Geometry check sheet. Reference: drawing and pictorial views, mm from the part's lowest x, y, z. Give positions to 0.01 mm unless a question says otherwise; leave off trailing zeros. Loops run counter-clockwise (first coordinate to the right, second up) from the corner with the lowest first, then second, coordinate; pieces in that order, holes last. Notation, with made-up numbers: (-12.75, 37.25) -> (10.25, 37.25) arc R16 ccw to (10.25, 41.25) -> close; hole circle Ø10 at (31.25, 6). An arc over 180 degrees is marked (long way). One line per item, written item: value. Start each with the question number.
(1) Gauge pin test, flat ends, axial feed: pin 1 Ø1 at (x, z) = (19, 0.5) entering from +Y; pin 2 Ø1.5 at (y, z) = (50.5, 1) entering from +X. Record the tip position at first contact, or that the pin passes through.
(2) Sectioned sample at B-B, the plane z = 0.75. Record the cut outline in (x, y), then the cut area to 3 significant figures.
(3) Sectioned sample at C-C, the plane y = 60. Record the cut outline in (x, z), then the cut area to 3 significant figures.
(4) Sectioned sample at D-D, the plane x = 48.5. Record the cut outline in (y, z).
(5) Scan lines: line 1 along X through (y, z) = (14.5, 1.9) (1 decimal); line 2 along Y through (x, z) = (15.5, 2.1) (1 decimal); line 3 along X through (y, z) = (72.5, 0.9) (1 decimal). Record each from-to range of solid material in increasing order. Write a range as from..to.
(6) Sectioned sample at A-A, the plane y = 15. Record the cut outline in (x, z), then the cut area to 3 significant figures.
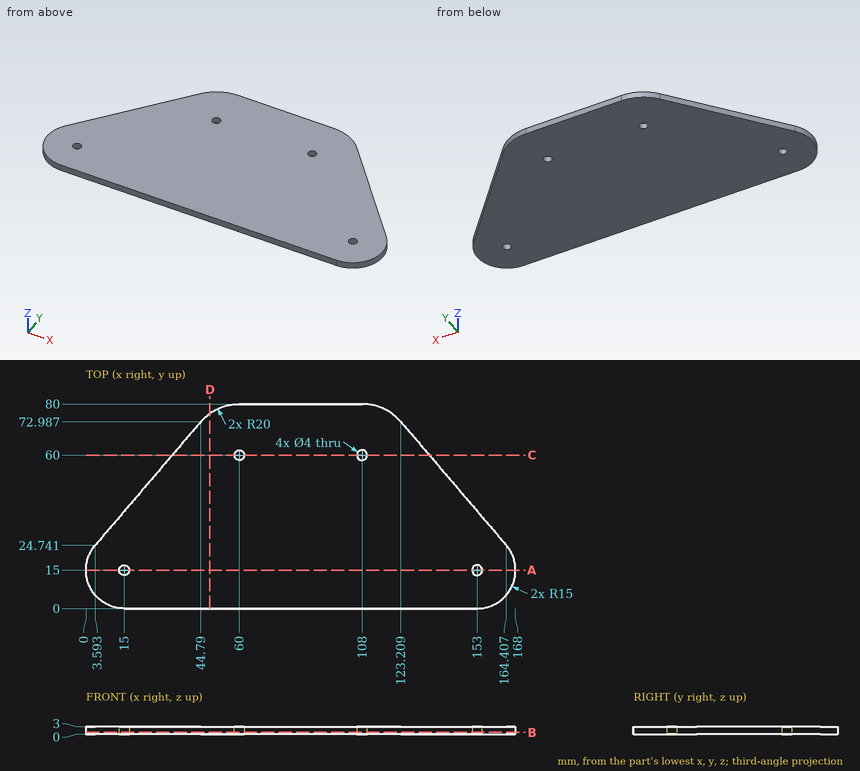
Calculated:
1. pin 1: stops at y = 43.37
1. pin 2: stops at x = 143.05
2. outline: (3.59, 24.74) arc R15 ccw to (15, 0) -> (153, 0) arc R15 ccw to (164.41, 24.74) -> (123.21, 72.99) arc R20 ccw to (108, 80) -> (60, 80) arc R20 ccw to (44.79, 72.99) -> close; hole circle Ø4 at (15, 15); hole circle Ø4 at (60, 60); hole circle Ø4 at (108, 60); hole circle Ø4 at (153, 15)
2. area: 10,200 mm2
3. outline: (33.7, 0) -> (58, 0) -> (58, 3) -> (33.7, 3) -> close; (62, 0) -> (106, 0) -> (106, 3) -> (62, 3) -> close; (110, 0) -> (134.3, 0) -> (134.3, 3) -> (110, 3) -> close
3. area: 278 mm2
4. outline: (0, 0) -> (76.36, 0) -> (76.36, 3) -> (0, 3) -> close
5. line 1: x = 0..13.1, 16.9..151.1, 154.9..168
5. line 2: y = 0..13.1, 16.9..38.7
5. line 3: x = 44.4..123.6
6. outline: (0, 0) -> (13, 0) -> (13, 3) -> (0, 3) -> close; (17, 0) -> (151, 0) -> (151, 3) -> (17, 3) -> close; (155, 0) -> (168, 0) -> (168, 3) -> (155, 3) -> close
6. area: 480 mm2
